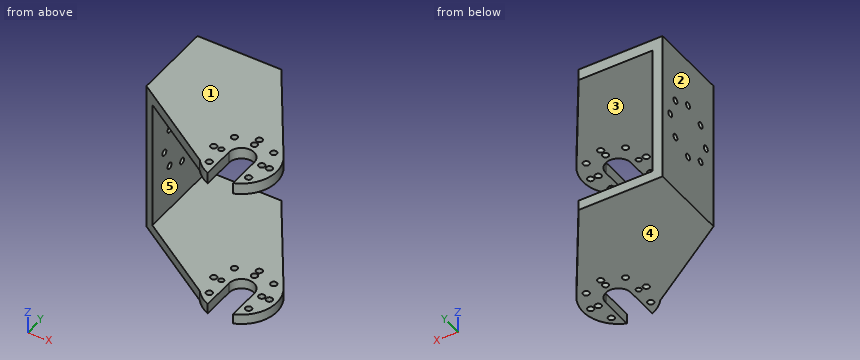
from build123d import *

# Parameters (mm, degrees)
SKETCH_1_R          = 5
SKETCH_1_R_2        = 1.225
SKETCH_1_R_3        = 1.025
EXTRUDE_1_DEPTH     = 60
SKETCH_2_W          = 57.132931415
SKETCH_2_H          = 51.5
CUT_EXTRUDE_1_DEPTH = 66
CUT_EXTRUDE_START   = -60.33903683
CUT_EXTRUDE_3_DEPTH = 60.33903683
SKETCH_8_R          = 1.225
CUT_EXTRUDE_4_DEPTH = 10


with BuildPart() as part:
    # 스케치1 → 보스-돌출1 (new body)
    with BuildSketch(Plane.XY):
        with BuildLine():
            Line((11.674013781, 7.727703555), (-14, 46.512678751))
            Line((-14, 46.512678751), (-47.132931415, 46.512678751))
            Line((-47.132931415, 46.512678751), (-47.132931415, 14.921692086))
            Line((-47.132931415, 14.921692086), (-11, -8.660254038))
            ThreePointArc((-11, -8.660254038), (8.200906179, -11.346591463), (11.674013781, 7.727703555))
        make_face()
        Circle(SKETCH_1_R, mode=Mode.SUBTRACT)
        with Locations((0, 8)):
            Circle(SKETCH_1_R_2, mode=Mode.SUBTRACT)
        with Locations((0, 11)):
            Circle(SKETCH_1_R_2, mode=Mode.SUBTRACT)
        with Locations((7.778174593, 7.778174593)):
            Circle(SKETCH_1_R_2, mode=Mode.SUBTRACT)
        with Locations((8, 0)):
            Circle(SKETCH_1_R_2, mode=Mode.SUBTRACT)
        with Locations((11, 0)):
            Circle(SKETCH_1_R_2, mode=Mode.SUBTRACT)
        with Locations((7.778174593, -7.778174593)):
            Circle(SKETCH_1_R_2, mode=Mode.SUBTRACT)
        with Locations((0, -8)):
            Circle(SKETCH_1_R_2, mode=Mode.SUBTRACT)
        with Locations((0, -11)):
            Circle(SKETCH_1_R_2, mode=Mode.SUBTRACT)
        with Locations((-7.778174593, -7.778174593)):
            Circle(SKETCH_1_R_2, mode=Mode.SUBTRACT)
        with Locations((-8, 0)):
            Circle(SKETCH_1_R_3, mode=Mode.SUBTRACT)
        with Locations((-11, 0)):
            Circle(SKETCH_1_R_2, mode=Mode.SUBTRACT)
        with Locations((-7.778174593, 7.778174593)):
            Circle(SKETCH_1_R_2, mode=Mode.SUBTRACT)
    extrude(amount=EXTRUDE_1_DEPTH)

    # 스케치2 → 컷-돌출1 (cut)
    with BuildSketch(Plane(origin=(0, 46.512678751, 0), x_dir=(1, 0, 0), z_dir=(0, 1, 0))):
        with Locations((-14.566465708, -29.75)):
            Rectangle(SKETCH_2_W, SKETCH_2_H)
    extrude(amount=-CUT_EXTRUDE_1_DEPTH, mode=Mode.SUBTRACT)

    # 스케치4 → 컷-돌출3 (cut)
    with BuildSketch(Plane.XY.offset(60).offset(CUT_EXTRUDE_START)):
        with BuildLine():
            Line((-5, 0), (-5, -13.076696831))
            ThreePointArc((-5, -13.076696831), (0, -14), (5, -13.076696831))
            Line((5, -13.076696831), (5, 0))
            Line((5, 0), (-5, 0))
        make_face()
    extrude(amount=CUT_EXTRUDE_3_DEPTH, mode=Mode.SUBTRACT)

    # 스케치8 → 컷-돌출4 (cut)
    with BuildSketch(Plane.ZY.offset(47.132931415)):
        with Locations(Location((22.217096027, 38.497340433, 0), (0, 0, 270))):
            Circle(SKETCH_8_R)
        with Locations(Location((29.99527062, 41.71916584, 0), (0, 0, 270))):
            Circle(SKETCH_8_R)
        with Locations(Location((37.773445213, 38.497340433, 0), (0, 0, 270))):
            Circle(SKETCH_8_R)
        with Locations(Location((40.99527062, 30.71916584, 0), (0, 0, 270))):
            Circle(SKETCH_8_R)
        with Locations(Location((37.773445213, 22.940991247, 0), (0, 0, 270))):
            Circle(SKETCH_8_R)
        with Locations(Location((29.99527062, 19.71916584, 0), (0, 0, 270))):
            Circle(SKETCH_8_R)
        with Locations(Location((22.217096027, 22.940991247, 0), (0, 0, 270))):
            Circle(SKETCH_8_R)
        with Locations(Location((18.99527062, 30.71916584, 0), (0, 0, 270))):
            Circle(SKETCH_8_R)
    extrude(amount=-CUT_EXTRUDE_4_DEPTH, mode=Mode.SUBTRACT)


solid = part.part
Model file for the job. Use its own axes, mm. Face numbers are marked on the shaded views. A direction names the side the tool comes from. Give positions to 0.01 mm unless a question says otherwise; leave off trailing zeros. Loops run counter-clockwise (first coordinate to the right, second up) from the corner with the lowest first, then second, coordinate; pieces in that order, holes last. Notation, with made-up numbers: (86.5, 40) -> (134.5, 40) arc R16 ccw to (134.5, 58) -> close; hole circle Ø5 at (29, 13.25). An arc over 180 degrees is marked (long way). Use a Markdown table: item, result. Add a question column.
(1) Slice it at B-B on x = 8. Give the number of separate pieces and of enclosed holes in the cut face, and give its area (3 significant figures).
(2) Mould opens along Z. For the marked faces 1, 2 and 3 say: +Z half, -Z half, draft (parallel to the pull), parting line (faces both ways), or undercut.
(3) Wall check: line 1 along Z through (x, y) = (-30, 40); line 2 along Y through (x, z) = (0, 1.25) (3 decimals); line 3 along X through (y, z) = (17.5, 26.5). Give the ranges that are in metal, low to high.
(4) Slice it at D-D on z = 54.5. List the corners of the cut face in (x, y), and give its area (3 significant figures).
(5) Slice it at A-A on x = -31.5. List the corners of the cut face in (y, z), and give its area (3 significant figures).
(6) Drop flat-ended pins along their axis: pin 1 Ø1.3 at (y, z) = (-9.5, 58.5) entering from +X; pin 2 Ø3 at (y, z) = (41.72, 30) entering from +X. Give the stop position or say it passes through.
(7) Slice it at C-C on y = 34. List the corners of the cut face in (x, z), and give its area (3 significant figures).
(8) Tool access for the marked faces 4 and 5: list every direction of +Z, -Z, +X, -X, +Y, -Y with a clear straight run to the whole face (end or side of a thin tool).
Filled sheet:
| question | item | result |
|---|---|---|
| 1 | separate pieces | 8 |
| 1 | enclosed holes | 0 |
| 1 | area | 149 mm2 |
| 2 | face 1 | +Z half |
| 2 | face 2 | draft |
| 2 | face 3 | undercut |
| 3 | line 1 | 0 to 4, 55.5 to 60 |
| 3 | line 2 | 5 to 6.775, 9.225 to 9.775, 12.225 to 25.363 |
| 3 | line 3 | -47.13 to -43.13 |
| 4 | outline | (-47.13, 14.92) -> (-43.13, 12.31) -> (-43.13, 46.51) -> (-47.13, 46.51) -> close |
| 4 | area | 132 mm2 |
| 5 | outline | (4.72, 0) -> (46.51, 0) -> (46.51, 4) -> (4.72, 4) -> close; (4.72, 55.5) -> (46.51, 55.5) -> (46.51, 60) -> (4.72, 60) -> close |
| 5 | area | 355 mm2 |
| 6 | pin 1 | x = 10.85 |
| 6 | pin 2 | x = -43.13 |
| 7 | outline | (-47.13, 0) -> (-5.72, 0) -> (-5.72, 4) -> (-43.13, 4) -> (-43.13, 55.5) -> (-5.72, 55.5) -> (-5.72, 60) -> (-47.13, 60) -> close |
| 7 | area | 558 mm2 |
| 8 | face 4 | -Z, +X, -X, +Y, -Y |
| 8 | face 5 | +X, +Y, -Y |
